CAD build for the part. Positions are in the model's coordinates, mm. Face numbers are marked on the shaded views. A direction names the side the tool comes from. Give positions to 0.01 mm unless a question says otherwise; leave off trailing zeros. Loops run counter-clockwise (first coordinate to the right, second up) from the corner with the lowest first, then second, coordinate; pieces in that order, holes last. Notation, with made-up numbers: (-30, -36.75) -> (-26, -36.75) arc R26 ccw to (-26, -4.75) -> close; hole circle Ø4 at (29, 34). An arc over 180 degrees is marked (long way). Use one line per item in the form item = value.
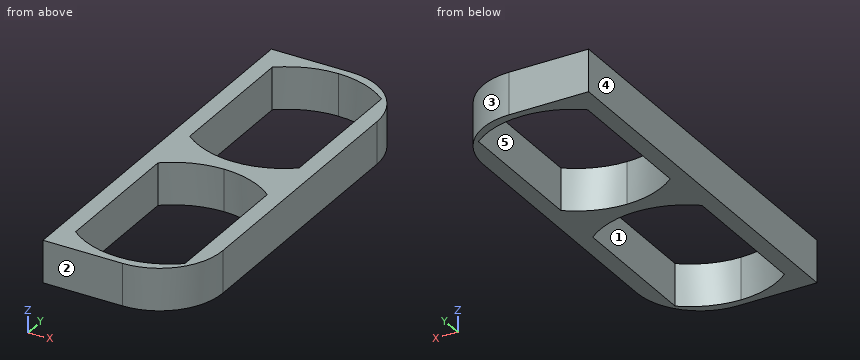
```python
from build123d import *

# Parameters (mm, degrees)
SKETCH1_W           = 47.5742
SKETCH1_H           = 58.42
BOSS_EXTRUDE1_DEPTH = 12.7
CUT_EXTRUDE1_REACH  = 41.753
SKETCH4_W           = 12.7
SKETCH4_H           = 116.84
CUT_EXTRUDE2_DEPTH  = 2.286
SKETCH5_W           = 12.7
SKETCH5_H           = 116.84
CUT_EXTRUDE3_DEPTH  = 2.286
FILLET1_R           = 19.05


with BuildPart() as part:
    # Sketch1 → Boss-Extrude1 (new body)
    with BuildSketch(Plane.XY):
        Rectangle(SKETCH1_W, SKETCH1_H)
    extrude(amount=BOSS_EXTRUDE1_DEPTH)

    # Sketch3 → Cut-Extrude1 (cut, up to next)
    with BuildSketch(Plane.XY.offset(12.7), mode=Mode.PRIVATE) as cut_extrude1_sk1:
        with BuildLine():
            ThreePointArc((-16.471621861, -21.087745183), (-8.737508184, -25.421809301), (0, -26.924))
            Line((0, -26.924), (0, 0))
            Line((0, 0), (0, 26.924))
            ThreePointArc((0, 26.924), (-8.737508184, 25.421809301), (-16.471621861, 21.087745183))
            Line((-16.471621861, 21.087745183), (-16.471621861, -21.087745183))
        make_face()
    cut_extrude1_tool1 = extrude(cut_extrude1_sk1.sketch, amount=-CUT_EXTRUDE1_REACH, mode=Mode.PRIVATE) & part.part
    # Sketch3 → Cut-Extrude1 (cut, up to next)
    with BuildSketch(Plane.XY.offset(12.7), mode=Mode.PRIVATE) as cut_extrude1_sk2:
        with BuildLine():
            Line((0, 0), (0, -26.924))
            ThreePointArc((0, -26.924), (8.737508184, -25.421809301), (16.471621861, -21.087745183))
            Line((16.471621861, -21.087745183), (16.471621861, 21.087745183))
            ThreePointArc((16.471621861, 21.087745183), (8.737508184, 25.421809301), (0, 26.924))
            Line((0, 26.924), (0, 0))
        make_face()
    cut_extrude1_tool2 = extrude(cut_extrude1_sk2.sketch, amount=-CUT_EXTRUDE1_REACH, mode=Mode.PRIVATE) & part.part
    add(cut_extrude1_tool1.solids().sort_by_distance((-7.924897, 0, 12.7))[0], mode=Mode.SUBTRACT)
    add(cut_extrude1_tool2.solids().sort_by_distance((7.924897, 0, 12.7))[0], mode=Mode.SUBTRACT)

    # Mirror1: part across plane


with BuildPart() as part_1:
    add(part.part)
    add(part.part.mirror(Plane(origin=(-23.7871, 29.21, 12.7), x_dir=(0, 0, 1), z_dir=(0, -1, 0))))

    # Sketch4 → Cut-Extrude2 (cut)
    with BuildSketch(Plane(origin=(23.7871, 0, 0), x_dir=(0, 0, -1), z_dir=(1, 0, 0))):
        with Locations((-6.35, 29.21)):
            Rectangle(SKETCH4_W, SKETCH4_H)
    extrude(amount=-CUT_EXTRUDE2_DEPTH, mode=Mode.SUBTRACT)

    # Sketch5 → Cut-Extrude3 (cut)
    with BuildSketch(Plane.ZY.offset(23.7871)):
        with Locations((6.35, 29.21)):
            Rectangle(SKETCH5_W, SKETCH5_H)
    extrude(amount=-CUT_EXTRUDE3_DEPTH, mode=Mode.SUBTRACT)

    # Fillet1
    fillet1_edges = [part_1.edges().sort_by_distance(p)[0] for p in [
        (21.5011, 87.63, 6.35),
        (21.5011, -29.21, 6.35),
    ]]
    fillet(fillet1_edges, radius=FILLET1_R)


solid = part_1.part
```
1. Drill centre lines: line 1 (Y direction, x = -1, z = 7); line 2 (X direction, y = 54.5, z = 6.75); line 3 (Y direction, x = -12.5, z = 6.25). Where is each one in solid material? Low to high.
Result sheet:
line_1 = -29.21 to -26.9, 26.9 to 31.52, 85.32 to 87.63
line_2 = -21.5 to -16.47, 16.47 to 21.5
line_3 = -29.21 to -23.74, 23.74 to 34.68, 82.16 to 87.63
2. Cut at A-A, the plane y = 67.5. Write the cut outline in (x, z), then the cut area to 3 significant figures.
Result sheet:
outline = (-21.5, 0) -> (-16.47, 0) -> (-16.47, 12.7) -> (-21.5, 12.7) -> close; (16.47, 0) -> (21.5, 0) -> (21.5, 12.7) -> (16.47, 12.7) -> close
area = 128 mm^2
3. Cut at D-D, the plane x = -10. Write the cut outline in (y, z), then the cut area to 3 significant figures.
Result sheet:
outline = (-29.21, 0) -> (-24.94, 0) -> (-24.94, 12.7) -> (-29.21, 12.7) -> close; (24.94, 0) -> (33.48, 0) -> (33.48, 12.7) -> (24.94, 12.7) -> close; (83.36, 0) -> (87.63, 0) -> (87.63, 12.7) -> (83.36, 12.7) -> close
area = 217 mm^2
4. Mould opens along X. For the marked faces 3, 4 and 5 say: pulls with the +X half, pulls with the -X half, needs draft (parallel to the pull), parting line crosses it, or undercut.
Result sheet:
face_3 = pulls with the +X half
face_4 = pulls with the -X half
face_5 = undercut
5. Cut at C-C, the plane z = 6.5. Write the cut outline in (x, y), then the cut area to 3 significant figures.
Result sheet:
outline = (-21.5, -29.21) -> (2.45, -29.21) arc R19.05 ccw to (21.5, -10.16) -> (21.5, 68.58) arc R19.05 ccw to (2.45, 87.63) -> (-21.5, 87.63) -> close; hole (-16.47, -21.09) arc R26.16 ccw to (16.47, -21.09) -> (16.47, 21.09) arc R26.16 ccw to (-16.47, 21.09) -> close; hole (-16.47, 37.33) arc R26.16 ccw to (16.47, 37.33) -> (16.47, 79.51) arc R26.16 ccw to (-16.47, 79.51) -> close
area = 1,560 mm^2
6. Tool access for the marked faces 1 and 2: list every direction of +Z, -Z, +X, -X, +Y, -Y with a clear straight run to the whole face (end or side of a thin tool).
Result sheet:
face_1 = +Z, -Z
face_2 = +Z, -Z, +X, -X, -Y
7. Cut at B-B, the plane x = 3.5. Write the cut outline in (y, z), then the cut area to 3 significant figures.
Result sheet:
outline = (-29.18, 0) -> (-26.69, 0) -> (-26.69, 12.7) -> (-29.18, 12.7) -> close; (26.69, 0) -> (31.73, 0) -> (31.73, 12.7) -> (26.69, 12.7) -> close; (85.11, 0) -> (87.6, 0) -> (87.6, 12.7) -> (85.11, 12.7) -> close
area = 127 mm^2
